from build123d import *

# Parameters (mm, degrees)
SKETCH1_R           = 28.575
EXTRUDE1_DEPTH      = 27.0002
EXTRUDE1_DEPTH_BACK = 84.1248
CUT_EXTRUDE1_REACH  = 86.125
SKETCH2_R           = 28.575
SKETCH2_R_2         = 23.622
CUT_EXTRUDE3_START  = -27.0002
CUT_EXTRUDE3_DEPTH  = 27.0002
SKETCH18_R          = 9.525
CUT_EXTRUDE4_DEPTH  = 0.254
SKETCH19_R          = 9.525
CUT_EXTRUDE5_DEPTH  = 0.254
CHAMFER1_SIZE       = 0.762
SKETCH15_R          = 6.9469
EXTRUDE2_DEPTH      = 1.27
CIRPATTERN1_COUNT   = 4


with BuildPart() as part:
    # Sketch1 → Extrude1 (new body, two sides)
    with BuildSketch(Plane(origin=(0, 0, 0), x_dir=(0, 0, -1), z_dir=(1, 0, 0))) as extrude1_sk:
        Circle(SKETCH1_R)
    extrude(amount=EXTRUDE1_DEPTH)
    extrude(extrude1_sk.sketch, amount=-EXTRUDE1_DEPTH_BACK)

    # Sketch2 → Cut-Extrude1 (cut, up to next)
    with BuildSketch(Plane(origin=(0, 0, 0), x_dir=(0, 0, -1), z_dir=(1, 0, 0)), mode=Mode.PRIVATE) as cut_extrude1_sk1:
        Circle(SKETCH2_R)
        with Locations((0, -4.191)):
            Circle(SKETCH2_R_2, mode=Mode.SUBTRACT)
    cut_extrude1_tool1 = extrude(cut_extrude1_sk1.sketch, amount=-CUT_EXTRUDE1_REACH, mode=Mode.PRIVATE) & part.part
    add(cut_extrude1_tool1.solids().sort_by_distance((0, 0, 27.766777))[0], mode=Mode.SUBTRACT)

    # Sketch4 → Cut-Extrude3 (cut)
    with BuildSketch(Plane.ZY.offset(CUT_EXTRUDE3_START)):
        with BuildLine():
            Line((23.6855, -25.666178421), (23.6855, 17.476089577))
            Line((23.6855, 17.476089577), (0, 31.150919378))
            Line((0, 31.150919378), (-23.6855, 17.476089577))
            Line((-23.6855, 17.476089577), (-23.6855, -25.666178421))
            ThreePointArc((-23.6855, -25.666178421), (0, 34.925), (23.6855, -25.666178421))
        make_face()
    extrude(amount=CUT_EXTRUDE3_DEPTH, mode=Mode.SUBTRACT)

    # Sketch6 → Cut-Revolve2 (revolve, cut)
    with BuildSketch(Plane.XY, mode=Mode.PRIVATE) as cut_revolve2_sk:
        Polygon((0.750392661, 57.15), (27.0002, 11.684), (27.0002, 57.15), align=None)
    revolve(cut_revolve2_sk.sketch.rotate(Axis((-0.562097706, -4.191, 0), (1, 0, 0)), 270), axis=Axis((-0.562097706, -4.191, 0), (1, 0, 0)), mode=Mode.SUBTRACT)  # turned: the seam where the file's is

    # S2D0002 → Cut-Revolve3 (revolve, cut)
    with BuildSketch(Plane(origin=(9.0932, 23.136869081, 13.372742289), x_dir=(0, 0.5, -0.866025404), z_dir=(1, 0, 0))):
        Polygon((0, 0), (6.1849, 0), (5.642306865, -2.5527), (4.9784, -3.216606865), (4.9784, -13.462), (0, -13.462), align=None)
    revolve(axis=Axis((9.0932, 10.895513396, 6.305192289), (0, 0.866025404, 0.5)), mode=Mode.SUBTRACT)

    # Sketch8 → Cut-Revolve4 (revolve, cut)
    with BuildSketch(Plane(origin=(9.0932, 23.136869081, -13.372742289), x_dir=(0, -0.5, -0.866025404), z_dir=(1, 0, 0))):
        Polygon((0, 0), (6.1849, 0), (5.642306865, -2.5527), (4.9784, -3.216606865), (4.9784, -13.462), (0, -13.462), align=None)
    revolve(axis=Axis((9.0932, 10.895513396, -6.305192289), (0, 0.866025404, -0.5)), mode=Mode.SUBTRACT)

    # Sketch18 → Cut-Extrude4 (cut)
    with BuildSketch(Plane(origin=(0, 23.363189534, 13.488743766), x_dir=(1, 0, 0), z_dir=(0, 0.866025404, 0.5))):
        with Locations((9.0932, -0.0127)):
            Circle(SKETCH18_R)
    extrude(amount=-CUT_EXTRUDE4_DEPTH, mode=Mode.SUBTRACT)

    # Sketch19 → Cut-Extrude5 (cut)
    with BuildSketch(Plane(origin=(0, 23.363189534, -13.488743766), x_dir=(1, 0, 0), z_dir=(0, 0.866025404, -0.5))):
        with Locations((9.0932, 0.0127)):
            Circle(SKETCH19_R)
    extrude(amount=-CUT_EXTRUDE5_DEPTH, mode=Mode.SUBTRACT)

    # Sketch10 → Cut-Revolve6 (revolve, cut)
    with BuildSketch(Plane.XY, mode=Mode.PRIVATE) as cut_revolve6_sk:
        Polygon((0, 19.431), (0, 18.415), (-3.302, 18.415), (-4.318, 19.431), align=None)
    revolve(cut_revolve6_sk.sketch.rotate(Axis((-4.5339, -4.191, 0), (1, 0, 0)), 90), axis=Axis((-4.5339, -4.191, 0), (1, 0, 0)), mode=Mode.SUBTRACT)  # turned: the seam where the file's is

    # Sketch12 → Cut-Revolve8 (revolve, cut)
    with BuildSketch(Plane.XY, mode=Mode.PRIVATE) as cut_revolve8_sk:
        Polygon((-84.1248, 19.431), (-84.1248, 18.415), (-81.5848, 18.415), (-80.5688, 19.431), align=None)
    revolve(cut_revolve8_sk.sketch.rotate(Axis((-84.3026, -4.191, 0), (1, 0, 0)), 90), axis=Axis((-84.3026, -4.191, 0), (1, 0, 0)), mode=Mode.SUBTRACT)  # turned: the seam where the file's is

    # Chamfer1
    chamfer1_edges = [part.edges().sort_by_distance(p)[0] for p in [
        (-84.1248, -4.191, -22.606),
    ]]
    chamfer(chamfer1_edges, length=CHAMFER1_SIZE)

    # Sketch13 → Revolve1 (revolve)
    with BuildSketch(Plane(origin=(0, 0, 0), x_dir=(0, -1, 0), z_dir=(0, 0, 1)), mode=Mode.PRIVATE) as revolve1_sk:
        with BuildLine():
            Line((4.191, 27.0002), (4.191, 64.8716))
            Line((4.191, 64.8716), (14.2875, 64.8716))
            ThreePointArc((14.2875, 64.8716), (15.00592049, 64.57402049), (15.3035, 63.8556))
            Line((15.3035, 63.8556), (15.3035, 27.0002))
            Line((15.3035, 27.0002), (4.191, 27.0002))
        make_face()
    revolve(revolve1_sk.sketch.rotate(Axis((25.10663, -4.191, 0), (1, 0, 0)), 270), axis=Axis((25.10663, -4.191, 0), (1, 0, 0)))  # turned: the seam where the file's is

    # S2D0001 → Cut-Revolve9 (revolve, cut)
    with BuildSketch(Plane(origin=(64.8716, -9.9441, 0), x_dir=(0, -1, 0), z_dir=(0, 0, 1)), mode=Mode.PRIVATE) as cut_revolve9_sk:
        Polygon((0, 0), (0, -17.018), (-5.7531, -20.474811227), (-5.7531, 0), align=None)
    revolve(cut_revolve9_sk.sketch.rotate(Axis((43.373048211, -4.191, 0), (1, 0, 0)), 270), axis=Axis((43.373048211, -4.191, 0), (1, 0, 0)), mode=Mode.SUBTRACT)  # turned: the seam where the file's is

    # Sketch15 → Extrude2 (add)
    with BuildSketch(Plane(origin=(27.0002, 23.143219081, -13.361743766), x_dir=(0, -0.5, -0.866025404), z_dir=(0, -0.866025404, 0.5))):
        with Locations((0.0127, -17.907)):
            Circle(SKETCH15_R)
    extrude(amount=-EXTRUDE2_DEPTH)

    # Sketch16 → Cut-Revolve10 (revolve, cut)
    with BuildSketch(Plane(origin=(60.9092, 3.666724106, -7.857724106), x_dir=(-1, 0, 0), z_dir=(0, -0.707106781, -0.707106781)), mode=Mode.PRIVATE) as cut_revolve10_sk:
        Polygon((0, 0), (2.413, 0), (0, -2.413), align=None)
    cut_revolve10 = revolve(cut_revolve10_sk.sketch.rotate(Axis((60.9092, 0.494324135, -4.685324135), (0, 0.707106781, -0.707106781)), 90), axis=Axis((60.9092, 0.494324135, -4.685324135), (0, 0.707106781, -0.707106781)), mode=Mode.SUBTRACT)  # turned: the seam where the file's is

    # CirPattern1: Cut-Revolve10 ×4 about axis
    cirpattern1_axis = Axis((25.10663, -4.191, 0), (-1, 0, 0))
    for i in range(1, CIRPATTERN1_COUNT):
        add(cut_revolve10.rotate(cirpattern1_axis, i * 360 / CIRPATTERN1_COUNT), mode=Mode.SUBTRACT)


solid = part.part
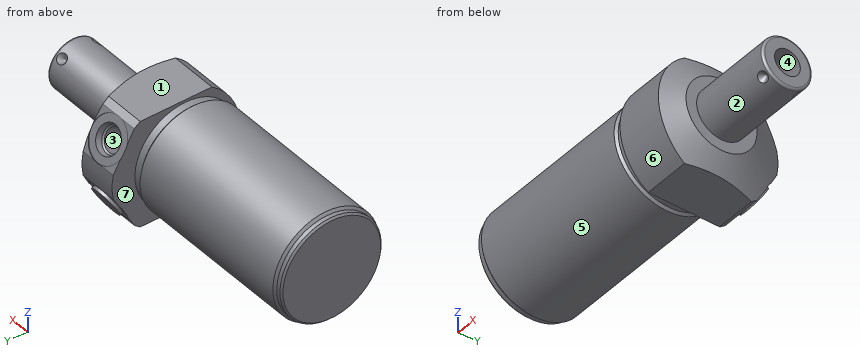
Geometry check sheet. Reference: the model listing, model coordinates, mm. Face numbers are marked on the shaded views. A direction names the side the tool comes from. Give positions to 0.01 mm unless a question says otherwise; leave off trailing zeros. Loops run counter-clockwise (first coordinate to the right, second up) from the corner with the lowest first, then second, coordinate; pieces in that order, holes last. Notation, with made-up numbers: M 7,22.25 L 38,22.25 A26 cw 38,41.25 Z; hole C -34.5,56.25 d10. An arc over 180 degrees is marked long. Write each question's results on one line, items separated by ' | '.
1) Tool access check on the marked faces 4, 5, 6 and 7. Record the directions out of +Z, -Z, +X, -X, +Y, -Y that give a thin tool (end or side, any length) a straight path to the whole face; none if there is none.
Answers follow:
face 4: +X | face 5: -X | face 6: +X, -X, -Y | face 7: none
2) Section check A-A, the plane x = -43. Record the boundary of the cut face in (y, z), plus the area to 3 significant figures.
Answers follow:
outline: C -4.19,0 d47.24 | area: 1,750 mm2
3) Thickness scan on line 1 (Z direction, x = 5.5, y = 11); line 2 (Y direction, x = 51.75, z = 0); line 3 (X direction, y = -13.5, z = 9). Record the ranges inside material, lowest first.
Answers follow:
line 1: -23.69 to -10.34, -7.47 to 7.47, 10.34 to 23.69 | line 2: -15.3 to -9.94, 1.56 to 6.92 | line 3: -84.12 to 27
4) Section check B-B, the plane x = 25.5. Record the boundary of the cut face in (y, z), plus the area to 3 significant figures.
Answers follow:
outline: C -4.19,0 d36.95 | area: 1,070 mm2
5) Gauge pin test, flat ends, axial feed: pin 1 (10 mm diameter, centred on y = -4, z = 13, fed in from +X); pin 2 (10 mm diameter, centred on x = -56.5, z = 18, fed in from +Y); pin 3 (10 mm diameter, centred on x = 2.5, z = 14.5, fed in from +Y); pin 4 (10 mm diameter, centred on y = 22.5, z = 8.5, fed in from +X). Record the tip position at first contact, or that the pin passes through.
Answers follow:
pin 1: x = 64.87 | pin 2: y = 15.53 | pin 3: y = 25.43 | pin 4: x = 22.88
6) Release check for a two-part mould opening along Y. For the marked faces 1, 2 and 3 record: +Y half, -Y half, draft (parallel to the pull), parting line (faces both ways), or undercut.
Answers follow:
face 1: draft | face 2: parting line | face 3: undercut
